```python
from build123d import *

# Parameters (mm, degrees)
F0_W     = 6.35
F0_H     = 292.1
F1_DEPTH = 457.2
F4_DEPTH = 304.801
F2_W     = 50.8
F2_H     = 190.5
F2_R     = 6.35
F5_DEPTH = 6.35
F6_W     = 31.75
F6_H     = 292.1
F7_DEPTH = 6.35


with BuildPart() as f1:
    # F0 (on Front) → F1 (new body)
    with BuildSketch(Plane.XZ):
        with BuildLine():
            Line((-139.7, -152.4), (139.7, -152.4))
            ThreePointArc((139.7, -152.4), (148.6802561211, -148.6802561211), (152.4, -139.7))
            Line((152.4, -139.7), (152.4, 139.7))
            ThreePointArc((152.4, 139.7), (148.6802561211, 148.6802561211), (139.7, 152.4))
            Line((139.7, 152.4), (-139.7, 152.4))
            ThreePointArc((-139.7, 152.4), (-148.6802561211, 148.6802561211), (-152.4, 139.7))
            Line((-152.4, 139.7), (-152.4, -139.7))
            ThreePointArc((-152.4, -139.7), (-148.6802561211, -148.6802561211), (-139.7, -152.4))
        make_face()
        with BuildLine():
            Line((0, 146.05), (139.7, 146.05))
            ThreePointArc((139.7, 146.05), (144.1901280605, 144.1901280605), (146.05, 139.7))
            Line((146.05, 139.7), (146.05, -139.7))
            ThreePointArc((146.05, -139.7), (144.1901280605, -144.1901280605), (139.7, -146.05))
            Line((139.7, -146.05), (0, -146.05))
            Line((0, -146.05), (-6.35, -146.05))
            Line((-6.35, -146.05), (-139.7, -146.05))
            ThreePointArc((-139.7, -146.05), (-144.1901280605, -144.1901280605), (-146.05, -139.7))
            Line((-146.05, -139.7), (-146.05, 139.7))
            ThreePointArc((-146.05, 139.7), (-144.1901280605, 144.1901280605), (-139.7, 146.05))
            Line((-139.7, 146.05), (-6.35, 146.05))
            Line((-6.35, 146.05), (0, 146.05))
        make_face(mode=Mode.SUBTRACT)
        with Locations((-3.175, 0)):
            Rectangle(F0_W, F0_H)
    extrude(amount=F1_DEPTH)

    # F3 (on face) → F4 (cut, through all)
    with BuildSketch(Plane(origin=(0, 0, -152.4), x_dir=(1, 0, 0), z_dir=(0, 0, -1))):
        Polygon((152.4, 143.4197438789), (152.4, 152.4), (139.7, 139.7), (139.7, 130.7197438789), align=None)
        Polygon((139.7, 130.7197438789), (139.7, 139.7), (0, 0), (8.9802561211, 0), align=None)
        Polygon((139.7, 0), (139.7, 130.7197438789), (8.9802561211, 0), align=None)
        Polygon((152.4, 0), (152.4, 143.4197438789), (139.7, 130.7197438789), (139.7, 0), align=None)
        Polygon((139.7, 365.1012237684), (139.7, 457.2), (-139.7, 457.2), (-139.7, 453.1957053812), align=None)
        Polygon((-139.7, 453.1957053812), (-139.7, 457.2), (-152.4, 457.2), align=None)
        Polygon((152.4, 361.0969291497), (152.4, 457.2), (139.7, 457.2), (139.7, 365.1012237684), align=None)
    extrude(amount=-F4_DEPTH, mode=Mode.SUBTRACT)

    # F2 (on face) → F5 (cut)
    with BuildSketch(Plane(origin=(0, 0, -152.4), x_dir=(1, 0, 0), z_dir=(0, 0, -1))):
        with Locations((73.025, 266.7)):
            Rectangle(F2_W, F2_H)
        with Locations((15.875, 171.45)):
            Circle(F2_R)
        with Locations((130.175, 171.45)):
            Circle(F2_R)
        with Locations((15.875, 361.95)):
            Circle(F2_R)
    extrude(amount=-F5_DEPTH, mode=Mode.SUBTRACT)

    # F6 (on face) → F7 (cut, through all)
    with BuildSketch(Plane(origin=(-6.35, 0, 0), x_dir=(0, -1, 0), z_dir=(-1, 0, 0))):
        with Locations((395.2756118842, 0)):
            Rectangle(F6_W, F6_H)
    extrude(amount=-F7_DEPTH, mode=Mode.SUBTRACT)


solid = f1.part
```
Verification items for the finished model (mm, model axes). A direction names the side the tool comes from. Coordinates: 2 decimals unless noted, no trailing zeros. Order: outer loops, then holes, each group sorted by start corner. A loop starts at its lowest first (then second) coordinate and runs counter-clockwise, first axis right, second up. Notation, with made-up numbers: (43.25, -11) -> (48.25, -11) arc R23 cw to (48.25, 23) -> close; hole circle Ø7 at (-20, 40.25). An arc over 180 degrees is marked (long way). Put each result on its own line as item: value. Start each with the question number.
1) Material ranges on L1, parallel to X at y = -324, z = 110; L2, parallel to Z at x = -70, y = -92.5; L3, parallel to X at y = -41, z = -42, recorded low to high.
2) Release check for a two-part mould opening along Z. For faces 1 (the cylindrical face through (-148.58, -225.4, 148.78)), 2 (the flat face through (-33, -223, 146.05)), 3 (the cylindrical face through (14.5, -355.75, -149.27)) record: pulls with the +Z half, pulls with the -Z half, needs draft (parallel to the pull), parting line crosses it, or undercut.
3) Cross-section at A-A (z = 52). Enter the section's corners in (x, y).
4) Tool access check on faces 4 (the flat face through (-6.35, -187, -2)), 5 (the cylindrical face through (19.289, -176.804, -149.269)), 6 (the flat face through (-3, 0, 46)). Record the directions out of +Z, -Z, +X, -X, +Y, -Y that give a thin tool (end or side, any length) a straight path to the whole face; none if there is none.
5) Cross-section at B-B (y = -116.5). Enter the section's corners in (x, z), plus the area to 3 significant figures.
6) Cross-section at C-C (x = -47.5). Enter the section's corners in (y, z), plus the area to 3 significant figures.
7) Cross-section at D-D (x = 15). Enter the section's corners in (y, z).
8) Go/stop test with flat-tipped pins: pin 1 (7 mm diameter, centred on x = -4, z = 66, fed in from -Y); pin 2 (2 mm diameter, centred on x = 67.5, y = -234, fed in from -Z); pin 3 (7 mm diameter, centred on x = 78, z = -149, fed in from +Y). Record where each tip stops, or that it passes through.
Geometry check:
1. L1: x = -152.4 to -146.05, -6.35 to 0, 146.05 to 152.4
1. L2: z = -152.4 to -146.05, 146.05 to 152.4
1. L3: x = -152.4 to -146.05, -6.35 to 0
2. face 1: pulls with the +Z half
2. face 2: undercut
2. face 3: needs draft
3. outline: (-152.4, -457.2) -> (-146.05, -455.2) -> (-146.05, 0) -> (-152.4, 0) -> close; (-6.35, -379.4) -> (0, -379.4) -> (0, 0) -> (-6.35, 0) -> close; (146.05, -363.1) -> (152.4, -361.1) -> (152.4, -152.4) -> (146.05, -146.05) -> close
4. face 4: +Y, -Y
4. face 5: -Z
4. face 6: +Z, -Z, +X, -X, +Y
5. outline: (-152.4, -139.7) arc R12.7 ccw to (-139.7, -152.4) -> (116.5, -152.4) -> (116.5, -146.05) -> (0, -146.05) -> (0, 146.05) -> (116.5, 146.05) -> (116.5, 152.4) -> (-139.7, 152.4) arc R12.7 ccw to (-152.4, 139.7) -> close; hole (-146.05, -139.7) arc R6.35 ccw to (-139.7, -146.05) -> (-6.35, -146.05) -> (-6.35, 146.05) -> (-139.7, 146.05) arc R6.35 ccw to (-146.05, 139.7) -> close
5. area: 7,070 mm^2
6. outline: (-424.13, -152.4) -> (0, -152.4) -> (0, -146.05) -> (-424.13, -146.05) -> close; (-424.13, 146.05) -> (0, 146.05) -> (0, 152.4) -> (-424.13, 152.4) -> close
6. area: 5,390 mm^2
7. outline: (-404.42, -152.4) -> (-368.24, -152.4) -> (-368.24, -146.05) -> (-404.42, -146.05) -> close; (-404.42, 146.05) -> (-15, 146.05) -> (-15, 152.4) -> (-404.42, 152.4) -> close; (-355.66, -152.4) -> (-177.74, -152.4) -> (-177.74, -146.05) -> (-355.66, -146.05) -> close; (-165.16, -152.4) -> (-15, -152.4) -> (-15, -146.05) -> (-165.16, -146.05) -> close
8. pin 1: stops at y = -379.4
8. pin 2: stops at z = 146.05
8. pin 3: stops at y = -74.5
